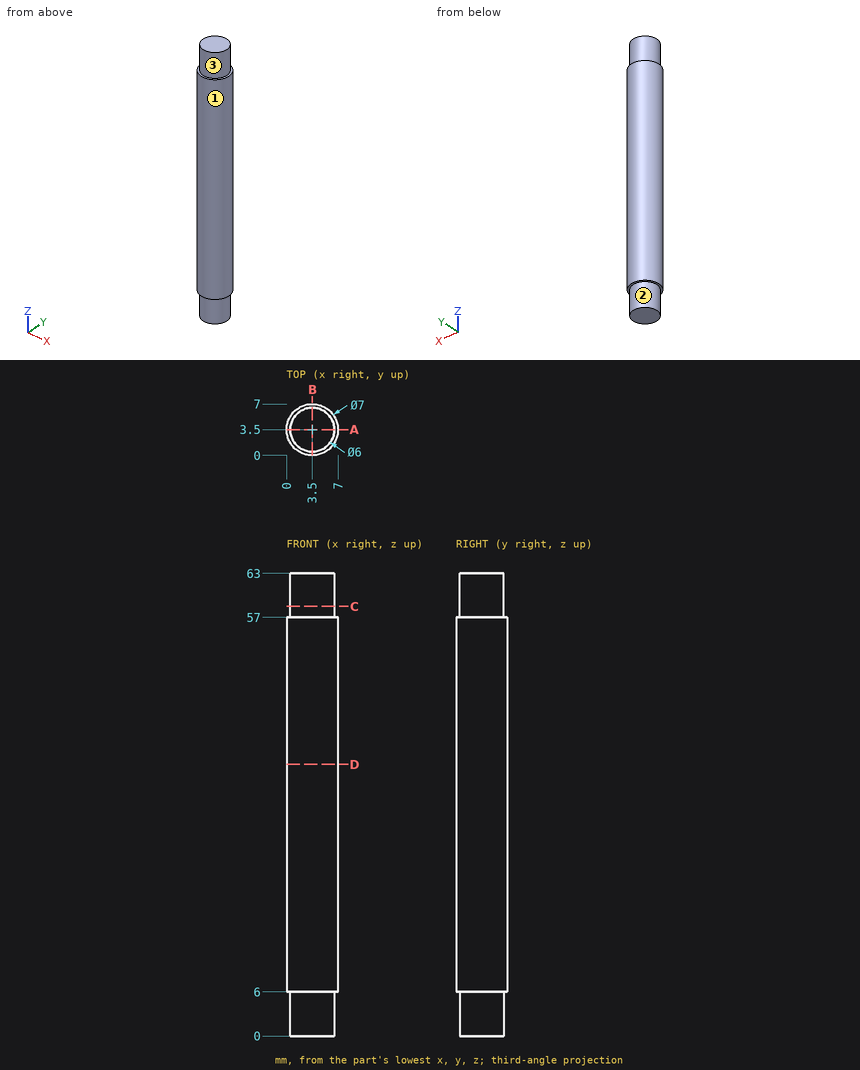
Design review of the part shown in the three views and the two pictorial views. Dimensions are in mm from the part's minimum x, y and z. A direction names the side the tool comes from. Round coordinates to 2 decimals unless told otherwise and drop trailing zeros. Write each loop counter-clockwise with the first axis right and the second up, starting at its lowest first coordinate (ties: lowest second). Pieces come first, ordered by that corner, then holes.
Item 1: Consider section A-A on y = 3.5. Give the boundary of the cut face in (x, z), and give its area (3 significant figures).
Item 2: For the marked faces 1, 2 and 3, list the 3-axis set-ups (+Z, -Z, +X, -X, +Y, -Y) from which the entire face can be reached by the end or side of a thin tool; tool diameter is ignored.
Item 3: Consider section D-D on z = 37. Give the boundary of the cut face in (x, y), and give its area (3 significant figures).
Item 4: Wall thickness on L1, parallel to Y at x = 3.75, z = 43.5; L2, parallel to Z at x = 0.5, y = 2.5: over which ranges is each line inside the solid? List them lowest first.
Item 5: Consider section C-C on z = 58.5. Give the boundary of the cut face in (x, y), and give its area (3 significant figures).
Check values:
1. outline: (0, 6) - (0.5, 6) - (0.5, 0) - (6.5, 0) - (6.5, 6) - (7, 6) - (7, 57) - (6.5, 57) - (6.5, 63) - (0.5, 63) - (0.5, 57) - (0, 57) - close
1. area: 429 mm2
2. face 1: +Z, -Z
2. face 2: -Z
2. face 3: +Z
3. outline: circle Ø7 at (3.5, 3.5)
3. area: 38.5 mm2
4. L1: y = 0.01 to 6.99
4. L2: z = 6 to 57
5. outline: circle Ø6 at (3.5, 3.5)
5. area: 28.3 mm2
